Check sheet for the modelled part. Datum: model origin and axes. Units: mm. A direction names the side the tool comes from. Coordinates: 2 decimals unless noted, no trailing zeros. Loops run counter-clockwise (first coordinate to the right, second up) from the corner with the lowest first, then second, coordinate; pieces in that order, holes last. Notation, with made-up numbers: M 80,0.25 L 104,0.25 A27 cw 104,18.25 Z; hole C -11,70.25 d1. An arc over 180 degrees is marked long. Write each question's results on one line, items separated by ' | '. Start each with the question number.
Autodesk Inventor part; units mm, degrees
ref_plane "YZ Plane" through (0, 0, 0) normal (1, 0, 0) x (0, 1, 0)
ref_plane "XZ Plane" through (0, 0, 0) normal (0, 1, 0) x (-1, 0, 0)
ref_plane "XY Plane" through (0, 0, 0) normal (0, 0, 1) x (1, 0, 0)
sketch "Boceto1" plane through (0, 0, 0) normal (0, 1, 0) x (-1, 0, 0)
  line L0 (140, 95) -> (-140, 95)
  line L1 (-140, 95) -> (-140, -95)
  line L2 (-140, -95) -> (140, -95)
  line L3 (140, -95) -> (140, 95)
  point P0 (0, 0)
  dimension "d0" = 280
  dimension "d1" = 190
  dimension "d2" = 95
  dimension "d3" = 140
extrude "Extrusión1" add sketch "Boceto1" along normal blind 130
ref_plane "Plano de trabajo1" through (0, 0, 95) normal (1, 0, 0) x (0, 0, -1)
ref_plane "Plano de trabajo2" through (140, 0, 0) normal (0, 0, -1) x (-1, 0, 0)
sketch "Boceto3" plane through (0, 130, 0) normal (0, 1, 0) x (1, 0, 0)
  line L0 (140, 95) -> (-140, 95)
  line L1 (-140, 95) -> (-140, -95)
  line L2 (-140, -95) -> (140, -95)
  line L3 (140, -95) -> (140, 95)
  line L4 (-135, -90) -> (135, -90)
  line L5 (135, -90) -> (135, 90)
  line L6 (135, 90) -> (-135, 90)
  line L7 (-135, 90) -> (-135, -90)
  point P0 (0, 0)
  dimension "d7" = 270
  dimension "d8" = 135
  dimension "d9" = 180
  dimension "d10" = 90
extrude "Extrusión2" cut sketch "Boceto3" against normal blind 125 contours L7 L6 L5 L4
sketch "Boceto4" plane through (-140, 0, -95) normal (-1, 0, 0) x (0, 0, 1)
  circle A0 centre (95, 29.1709) radius 10
  point P0 (95, 0)
  dimension "d13" = 20
extrude "Extrusión3" cut sketch "Boceto4" against normal blind 5
sketch "Boceto6" plane through (0, 130, 0) normal (0, 1, 0) x (1, 0, 0)
  line L0 (-140, -95) -> (140, -95)
  line L1 (-140, 95) -> (-140, -95)
  line L2 (140, 95) -> (-140, 95)
  line L3 (140, -95) -> (140, 95)
  line L4 (-140, -95) -> (140, -95)
  line L5 (140, -95) -> (140, 95)
  line L6 (140, 95) -> (-140, 95)
  line L7 (-140, 95) -> (-140, -95)
  point P0 (0, 0)
extrude "Extrusión4" [suppressed]
properties part number "cajaEléctrica"
1) Release check for a two-part mould opening along X. For faces 4 (the flat face through (135, 68, 1)), 5 (the flat face through (-140, 64, -1)), 6 (the flat face through (140, 64, 1)), 7 (the flat face through (-2, 64, 95)) record: +X half, -X half, draft (parallel to the pull), parting line (faces both ways), or undercut.
2) Section check D-D (x = 21.5). Enter the section's corners in (y, z).
3) Gauge pin test, flat end, axial feed: P1, Ø10, axis at x = 21, z = -3.5, coming from the +Y side. Record the tip position at first contact, or that the pin passes through.
4) Thickness scan on probe 1 along Y at (x, z) = (-136.25, 0); probe 2 along Z at (x, y) = (-77.5, 17); probe 3 along X at (y, z) = (22.5, 40.5). Record the ranges inside material, lowest first.
5) Section check A-A (z = 0). Enter the section's corners in (x, y).
6) Section check B-B (y = 88.5). Enter the section's corners in (x, z), then the cut area to 3 significant figures.
7) Set-up check for faces 1 (the cylindrical face through (-137.54, 37.6, 5.38)), 2 (the flat face through (2, 0, 1)), 3 (the flat face through (2, 68, -90)): record each of +Z, -Z, +X, -X, +Y, -Y from which the full face is reachable in a straight line by a thin tool's end or side.
8) Section check C-C (z = 72). Enter the section's corners in (x, y).
Return value:
1) face 4: undercut | face 5: -X half | face 6: +X half | face 7: draft
2) outline: M 0,-95 L 130,-95 L 130,-90 L 5,-90 L 5,90 L 130,90 L 130,95 L 0,95 Z
3) P1: stops at y = 5
4) probe 1: y = 0 to 19.17, 39.17 to 130 | probe 2: z = -95 to -90, 90 to 95 | probe 3: x = -140 to -135, 135 to 140
5) outline: M -140,0 L 140,0 L 140,130 L 135,130 L 135,5 L -135,5 L -135,19.17 L -140,19.17 Z; M -140,39.17 L -135,39.17 L -135,130 L -140,130 Z
6) outline: M -140,-95 L 140,-95 L 140,95 L -140,95 Z; hole M -135,-90 L 135,-90 L 135,90 L -135,90 Z | area: 4,600 mm2
7) face 1: -X | face 2: +Z, -Z, +X, -X, -Y | face 3: +Y
8) outline: M -140,0 L 140,0 L 140,130 L 135,130 L 135,5 L -135,5 L -135,130 L -140,130 Z
